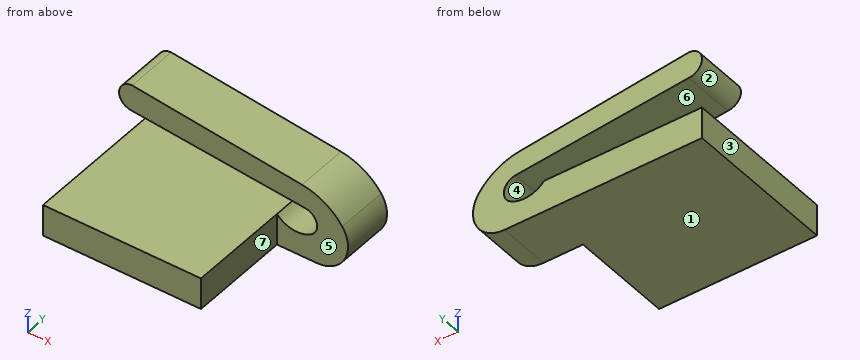
from build123d import *

# Parameters (mm, degrees)
BOSS_EXTRUDE1_DEPTH = 2
SKETCH2_W           = 6
SKETCH2_H           = 1.2
BOSS_EXTRUDE2_DEPTH = 3.9
FILLET1_DEPTH       = 2


with BuildPart() as part:
    # Sketch1 → Boss-Extrude1 (new body)
    with BuildSketch(Plane(origin=(0, 0, 0), x_dir=(1, 0, 0), z_dir=(0, 1, 0))):
        with BuildLine():
            Line((0, 1.2), (7.5, 1.2))
            ThreePointArc((7.5, 1.2), (8.567707825, 0.547722558), (8.474679434, -0.7))
            ThreePointArc((8.474679434, -0.7), (7.807430734, -1.311314361), (6.951049145, -1.603780854))
            Line((6.951049145, -1.603780854), (0.5, -2.4))
            ThreePointArc((0.5, -2.4), (0, -1.9), (0.5, -1.4))
            Line((0.5, -1.4), (7.5, -0.7))
            ThreePointArc((7.5, -0.7), (7.642928579, -0.35), (7.5, 0))
            ThreePointArc((7.5, 0), (6.75, 0.338562172), (6, 0))
            Line((6, 0), (0, 0))
            Line((0, 0), (0, 1.2))
        make_face()
    extrude(amount=BOSS_EXTRUDE1_DEPTH)

    # Sketch2 → Boss-Extrude2 (add)
    with BuildSketch(Plane(origin=(0, 0, 0), x_dir=(1, 0, 0), z_dir=(0, 1, 0))):
        with Locations((3, 0.6)):
            Rectangle(SKETCH2_W, SKETCH2_H)
    extrude(amount=-BOSS_EXTRUDE2_DEPTH)

    # Fillet1: read off the stored shape, not the designer's step
    # Fillet1 outline → Fillet1 (add)
    with BuildSketch(Plane(origin=(0, 0, 0), x_dir=(1, 0, 0), z_dir=(0, 1, 0))):
        with BuildLine():
            ThreePointArc((7.5, 0), (7.407145524, 0.092325902), (7.303023614, 0.171727751))
            ThreePointArc((7.303023614, 0.171727751), (7.511802782, -0.365240542), (7.076263667, -0.742373633))
            Line((7.076263667, -0.742373633), (7.5, -0.7))
            ThreePointArc((7.5, -0.7), (7.642928579, -0.35), (7.5, 0))
        make_face()
    extrude(amount=FILLET1_DEPTH)


solid = part.part
Read the model definition and answer for the solid it produces. Units are mm, in the model's axes. Face numbers are marked on the shaded views. A direction names the side the tool comes from. Coordinates: 2 decimals unless noted, no trailing zeros. Write each loop counter-clockwise with the first axis right and the second up, starting at its lowest first coordinate (ties: lowest second). Pieces come first, ordered by that corner, then holes. Notation, with made-up numbers: (41.5, 65) - (71.5, 65) arc R35 ccw to (71.5, 99) - close; hole circle Ø2 at (45.5, 12.25). An arc over 180 degrees is marked (long way). One line per question, with ' | ' between items.
Q1. Find section B-B, the plane y = -2.5. Write down the section's boundary in (x, z).
Result set:
outline: (0, -1.2) - (6, -1.2) - (6, 0) - (0, 0) - close
Q2. Find section C-C, the plane z = 1.7. Write down the section's boundary in (x, y).
Result set:
outline: (0.04, 0) - (6.17, 0) - (6.17, 2) - (0.04, 2) - close
Q3. Consider L1, parallel to Z at x = 4.25, y = -3.55; L2, parallel to X at y = -2.15, z = -0.35; L3, parallel to Y at x = 8, z = -0.95. Determine where each line is inside the solid, lowest interval first. Write a range as [from, to].
Result set:
L1: [-1.2, 0] | L2: [0, 6] | L3: [0, 2]
Q4. Determine the mould class of the marked faces 1, 2 and 3 for opening direction Z: +Z half, -Z half, draft (parallel to the pull), parting line (faces both ways), or undercut.
Result set:
face 1: -Z half | face 2: undercut | face 3: draft
Q5. Find section A-A, the plane x = 5. Write down the section's boundary in (y, z), plus the area to 3 significant figures.
Result set:
outline: (-3.9, -1.2) - (2, -1.2) - (2, 0) - (-3.9, 0) - close; (0, 0.95) - (2, 0.95) - (2, 1.84) - (0, 1.84) - close | area: 8.87 mm^2
Q6. Each of these flat-tipped pins is pushed along its axis until it touches: P1, Ø1.3, axis at y = -3, z = -0.5, coming from the +X side; P2, Ø3, axis at x = 4, y = -2, coming from the +Z side. Where does it stop, or does it pass through?
Result set:
P1: x = 6 | P2: z = 0
Q7. For the marked faces 4, 5, 6 and 7, determine the directions among +Z, -Z, +X, -X, +Y, -Y from which every point of the face is accessible in a straight line to the end or side of a thin tool.
Result set:
face 4: +Y, -Y | face 5: +Z, +X, -Y | face 6: -X, +Y, -Y | face 7: +Z, -Z, +X, -Y
